```python
from build123d import *

# Parameters (mm, degrees)
SKETCH1_R               = 2.413
EXTRUDE1_DEPTH          = 77.6605
SKETCH8_OUTSIDE_W       = 305.288
SKETCH8_OUTSIDE_H       = 307.252
SKETCH8_OUTSIDE_R       = 6.35
EXTRUDE4_DEPTH          = 79.26390671
EXTRUDE4_DRAFT          = -60
MIRROR1_COPY_1_SKETCH_W = 305.288
MIRROR1_COPY_1_SKETCH_H = 307.252
MIRROR1_COPY_1_SKETCH_R = 6.35
MIRROR1_COPY_1_DEPTH    = 79.26390671
MIRROR1_COPY_1_DRAFT    = -60
BOSS_EXTRUDE1_START     = -5.08
SKETCH13_R              = 6.35
SKETCH13_R_2            = 2.413
BOSS_EXTRUDE1_DEPTH     = 5.08


with BuildPart() as part:
    # Sketch1 → Extrude1 (new body)
    with BuildSketch(Plane.XY):
        Polygon((0, 7.332348419), (-6.35, 3.666174209), (-6.35, -3.666174209), (0, -7.332348419), (6.35, -3.666174209), (6.35, 3.666174209), align=None)
        Circle(SKETCH1_R, mode=Mode.SUBTRACT)
    extrude(amount=EXTRUDE1_DEPTH)

    # Extrude3 cone 1 section (through the dimple's axis) → Extrude3 (revolve, cut)
    with BuildSketch(Plane.YZ):
        Polygon((0, 0), (2.4638, 0), (0, 2.642102028), align=None)
    revolve(axis=Axis((0, 0, 0), (0, 0, 1)), mode=Mode.SUBTRACT)


with BuildPart() as extrude4_tool:
    # Sketch8 outside → Extrude4 (with draft: the straight prism first)
    with BuildSketch(Plane(origin=(0, 0, 0), x_dir=(-1, 0, 0), z_dir=(0, 0, -1))):
        Rectangle(SKETCH8_OUTSIDE_W, SKETCH8_OUTSIDE_H)
        Circle(SKETCH8_OUTSIDE_R, mode=Mode.SUBTRACT)
    extrude(amount=-EXTRUDE4_DEPTH)
    # Extrude4: the draft: its side faces are tilted about the plane it starts from
    extrude4_sides = [extrude4_tool.faces().sort_by_distance(p)[0] for p in [
        (0, -153.626, 39.631953355),
        (-152.644, 0, 39.631953355),
        (0, 153.626, 39.631953355),
        (152.644, 0, 39.631953355),
        (6.35, 0, 39.631953355),
    ]]
    draft(extrude4_sides, Plane(origin=(0, 0, 0), x_dir=(-1, 0, 0), z_dir=(0, 0, -1)), EXTRUDE4_DRAFT)


with BuildPart() as part_1:
    add(part.part)

    # Extrude4: cut by extrude4_tool
    add(extrude4_tool.part, mode=Mode.SUBTRACT)


with BuildPart() as mirror1_copy_1_tool:
    # Mirror1 copy 1 sketch → Mirror1 copy 1 (with draft: the straight prism first)
    with BuildSketch(Plane(origin=(0, 0, 77.6605), x_dir=(-1, 0, 0), z_dir=(0, 0, 1))):
        Rectangle(MIRROR1_COPY_1_SKETCH_W, MIRROR1_COPY_1_SKETCH_H)
        Circle(MIRROR1_COPY_1_SKETCH_R, mode=Mode.SUBTRACT)
    extrude(amount=-MIRROR1_COPY_1_DEPTH)
    # Mirror1 copy 1: the draft: its side faces are tilted about the plane it starts from
    mirror1_copy_1_sides = [mirror1_copy_1_tool.faces().sort_by_distance(p)[0] for p in [
        (0, -153.626, 38.028546645),
        (-152.644, 0, 38.028546645),
        (0, 153.626, 38.028546645),
        (152.644, 0, 38.028546645),
        (6.35, 0, 38.028546645),
    ]]
    draft(mirror1_copy_1_sides, Plane(origin=(0, 0, 77.6605), x_dir=(-1, 0, 0), z_dir=(0, 0, 1)), MIRROR1_COPY_1_DRAFT)


with BuildPart() as part_2:
    add(part_1.part)

    # Mirror1 copy 1: cut by mirror1_copy_1_tool
    add(mirror1_copy_1_tool.part, mode=Mode.SUBTRACT)

    # Sketch13 → Boss-Extrude1 (add)
    with BuildSketch(Plane.XY.offset(BOSS_EXTRUDE1_START)):
        Circle(SKETCH13_R)
        with Locations(Location((0, 0, 0), (0, 0, 180))):
            Circle(SKETCH13_R_2, mode=Mode.SUBTRACT)
    extrude(amount=BOSS_EXTRUDE1_DEPTH)


solid = part_2.part
```
Input: part model. Units: mm. Frame: model coordinates. A direction names the side the tool comes from. Round coordinates to 2 decimals unless told otherwise and drop trailing zeros. Loops run counter-clockwise (first coordinate to the right, second up) from the corner with the lowest first, then second, coordinate; pieces in that order, holes last. Notation, with made-up numbers: (7.5, 66.5) -> (44.5, 66.5) arc R26 ccw to (44.5, 91.5) -> close; hole circle Ø4 at (34, -25). An arc over 180 degrees is marked (long way). Use one line per item in the form item = value. Start each with the question number.
Item 1: Material intervals for L1, parallel to X at y = 0, z = 34; L2, parallel to Y at x = 0, z = 22; L3, parallel to Y at x = 4.25, z = 18.5, sorted ascending. Write a range as from..to.
Item 2: Mould query, pull axis X, two halves, no side actions, for faces 3 (the face through (-0.016, 6.584, 0.135)), 4 (the face through (-3.219, -5.474, 38.287)), 5 (the face through (-1.915, -1.468, 38.314)). Classes: pulls with the +X half, pulls with the -X half, needs draft (parallel to the pull), parting line crosses it, or undercut.
Item 3: Set-up query: faces 1 (the face through (-1.38, -6.2, -2.58)), 2 (the face through (3, 0, 77.66)). Return all of +Z, -Z, +X, -X, +Y, -Y with unobstructed straight access to the full face (end or side cutting, diameter ignored); none if empty.
Item 4: Section query A-A on z = 17. Return the cut outline in (x, y).
Item 5: Contact query for flat-ended pins moving along their axis: pin 1 Ø4.5 at (x, y) = (0, 0) entering from -Z; pin 2 Ø2 at (y, z) = (4.5, 14) entering from -X; pin 3 Ø1.5 at (x, z) = (2.5, 20.5) entering from +Y. Output: stop coordinate, or through.
Ans:
q1.L1 = -6.35..-2.41, 2.41..6.35
q1.L2 = -7.33..-2.41, 2.41..7.33
q1.L3 = -4.88..4.88
q2.face_3 = parting line crosses it
q2.face_4 = pulls with the -X half
q2.face_5 = undercut
q3.face_1 = -Z
q3.face_2 = +Z, +X, -X, +Y, -Y
q4.outline = (-6.35, -3.67) -> (0, -7.33) -> (6.35, -3.67) -> (6.35, 3.67) -> (0, 7.33) -> (-6.35, 3.67) -> close; hole circle Ø4.83 at (0, 0)
q5.pin_1 = through
q5.pin_2 = -6.35
q5.pin_3 = 6.32
